```python
from build123d import *

# Parameters (mm, degrees)
SKETCH1_R               = 20
SKETCH1_R_2             = 7.5
BOSS_EXTRUDE1_DEPTH     = 36.5
SKETCH4_R               = 51.5
CUT_EXTRUDE3_DEPTH      = 31.5
CUT_EXTRUDE4_DEPTH      = 247.841548367
CUT_EXTRUDE4_DEPTH_BACK = 247.841548367
SKETCH5_W               = 26.5
SKETCH5_H               = 90
SHELL1_START            = 6
SHELL1_DEPTH            = 30.5
BOSS_EXTRUDE2_START     = -7.5
SKETCH7_R               = 2
BOSS_EXTRUDE2_DEPTH     = 7.5
BOSS_EXTRUDE3_DEPTH     = 15
CUT_EXTRUDE5_DEPTH      = 247.025913269
CUT_EXTRUDE5_DEPTH_BACK = 6
SKETCH9_R               = 5
SKETCH9_R_2             = 1.5
CUT_EXTRUDE6_DEPTH      = 6
FILLET1_R               = 10
SKETCH11_R              = 1.55
CUT_EXTRUDE7_DEPTH      = 247.841548367
SKETCH12_R              = 3.55
CUT_EXTRUDE8_DEPTH      = 3
SKETCH13_R              = 12.1
CUT_EXTRUDE9_DEPTH      = 5


# Read off the part's stored shape, not the designer's step: Shell1
with BuildPart() as part:
    # Sketch1 → Boss-Extrude1 (new body)
    with BuildSketch(Plane.XY):
        with BuildLine():
            ThreePointArc((-54.352625843, 15.42861186), (0, -56.5), (54.352625843, 15.42861186))
            ThreePointArc((54.352625843, 15.42861186), (37.535595393, 105.258460348), (37.34995219, 196.64872093))
            ThreePointArc((37.34995219, 196.64872093), (0, 237.5), (-37.34995219, 196.64872093))
            ThreePointArc((-37.34995219, 196.64872093), (-37.535595393, 105.258460348), (-54.352625843, 15.42861186))
        make_face()
        Circle(SKETCH1_R, mode=Mode.SUBTRACT)
        with Locations((0, 200)):
            Circle(SKETCH1_R_2, mode=Mode.SUBTRACT)
    extrude(amount=BOSS_EXTRUDE1_DEPTH)

    # Sketch4 → Cut-Extrude3 (cut)
    with BuildSketch(Plane.XY.offset(36.5)):
        Circle(SKETCH4_R)
    extrude(amount=-CUT_EXTRUDE3_DEPTH, mode=Mode.SUBTRACT)

    # Sketch5 → Cut-Extrude4 (cut, two sides: drawn at the far end of the back side and taken through both)
    with BuildSketch(Plane(origin=(0, 0, 0), x_dir=(0, 0, -1), z_dir=(1, 0, 0)).offset(-CUT_EXTRUDE4_DEPTH_BACK)):
        with Locations((-23.25, 192.5)):
            Rectangle(SKETCH5_W, SKETCH5_H)
    extrude(amount=CUT_EXTRUDE4_DEPTH + CUT_EXTRUDE4_DEPTH_BACK, mode=Mode.SUBTRACT)

    # Shell1 outline → Shell1 (cut)
    with BuildSketch(Plane.XY.offset(SHELL1_START)):
        with BuildLine():
            ThreePointArc((-42.077009937, 39.188968279), (0, 57.5), (42.077009937, 39.188968279))
            ThreePointArc((42.077009937, 39.188968279), (33.155030313, 90.022278833), (29.457543912, 141.5))
            Line((29.457543912, 141.5), (-29.457543912, 141.5))
            ThreePointArc((-29.457543912, 141.5), (-33.155030313, 90.022278833), (-42.077009937, 39.188968279))
        make_face()
    extrude(amount=SHELL1_DEPTH, mode=Mode.SUBTRACT)

    # Sketch7 → Boss-Extrude2 (add)
    # profile 1 of 2: a face of its own
    with BuildSketch(Plane.XY.offset(36.5).offset(BOSS_EXTRUDE2_START)):
        with BuildLine():
            Line((-39.159181835, 90.358571571), (-46.159181835, 97.5))
            Line((-46.159181835, 97.5), (-46.159181835, 112.5))
            Line((-46.159181835, 112.5), (-36.669554937, 115.653883533))
            ThreePointArc((-36.669554937, 115.653883533), (-37.753606302, 102.990404952), (-39.159181835, 90.358571571))
        make_face()
        with Locations((-42.159181835, 105)):
            Circle(SKETCH7_R, mode=Mode.SUBTRACT)
    # profile 2 of 2: a face of its own
    with BuildSketch(Plane.XY.offset(36.5).offset(BOSS_EXTRUDE2_START)):
        with BuildLine():
            Line((46.159181835, 97.5), (46.159181835, 112.5))
            Line((46.159181835, 112.5), (36.669554937, 115.653883533))
            ThreePointArc((36.669554937, 115.653883533), (37.753606302, 102.990404952), (39.159181835, 90.358571571))
            Line((39.159181835, 90.358571571), (46.159181835, 97.5))
        make_face()
        with Locations(Location((42.159181835, 105, 0), (0, 0, 180))):
            Circle(SKETCH7_R, mode=Mode.SUBTRACT)
    extrude(amount=BOSS_EXTRUDE2_DEPTH)

    # Sketch8 → Boss-Extrude3 (add)
    with BuildSketch(Plane.XY.offset(6)):
        with BuildLine():
            Line((-35.707844492, 72), (-25.707844492, 72))
            Line((-25.707844492, 72), (-25.707844492, 69.5))
            Line((-25.707844492, 69.5), (-36.114376268, 69.5))
            ThreePointArc((-36.114376268, 69.5), (-35.909546125, 70.749745632), (-35.707844492, 72))
        make_face()
        with BuildLine():
            Line((-36.705134195, 66), (-25.707844492, 66))
            Line((-25.707844492, 66), (-25.707844492, 63))
            Line((-25.707844492, 63), (-37.231629056, 63))
            ThreePointArc((-37.231629056, 63), (-36.966124321, 64.499603847), (-36.705134195, 66))
        make_face()
        with BuildLine():
            Line((25.707844492, 63), (37.231629056, 63))
            ThreePointArc((37.231629056, 63), (36.966124321, 64.499603847), (36.705134195, 66))
            Line((36.705134195, 66), (25.707844492, 66))
            Line((25.707844492, 66), (25.707844492, 63))
        make_face()
        with BuildLine():
            Line((25.707844492, 69.5), (36.114376268, 69.5))
            ThreePointArc((36.114376268, 69.5), (35.909546125, 70.749745632), (35.707844492, 72))
            Line((35.707844492, 72), (25.707844492, 72))
            Line((25.707844492, 72), (25.707844492, 69.5))
        make_face()
    extrude(amount=BOSS_EXTRUDE3_DEPTH)

    # Sketch9 → Cut-Extrude5 (cut, two sides: drawn at the far end of the back side and taken through both)
    with BuildSketch(Plane.XY.offset(6).offset(-CUT_EXTRUDE5_DEPTH_BACK)):
        with Locations((0, 90.5)):
            Circle(SKETCH9_R)
        with Locations((-15.5, 106)):
            Circle(SKETCH9_R_2)
        with Locations((15.5, 106)):
            Circle(SKETCH9_R_2)
        with Locations((15.5, 75)):
            Circle(SKETCH9_R_2)
        with Locations((-15.5, 75)):
            Circle(SKETCH9_R_2)
    extrude(amount=CUT_EXTRUDE5_DEPTH + CUT_EXTRUDE5_DEPTH_BACK, mode=Mode.SUBTRACT)

    # Sketch10 → Cut-Extrude6 (cut)
    with BuildSketch(Plane.XY.offset(6)):
        with BuildLine():
            Line((-13.327049627, 124), (-1.672950373, 124))
            ThreePointArc((-1.672950373, 124), (-0.48999582, 123.51000418), (0, 122.327049627))
            Line((0, 122.327049627), (0, 122.172950373))
            ThreePointArc((0, 122.172950373), (-0.48999582, 120.98999582), (-1.672950373, 120.5))
            Line((-1.672950373, 120.5), (-13.327049627, 120.5))
            ThreePointArc((-13.327049627, 120.5), (-14.51000418, 120.98999582), (-15, 122.172950373))
            Line((-15, 122.172950373), (-15, 122.327049627))
            ThreePointArc((-15, 122.327049627), (-14.51000418, 123.51000418), (-13.327049627, 124))
        make_face()
    extrude(amount=-CUT_EXTRUDE6_DEPTH, mode=Mode.SUBTRACT)

    # Fillet1
    fillet1_edges = [part.edges().sort_by_distance(p)[0] for p in [
        (35.369251346, 147.5, 23.25),
        (-35.369251346, 147.5, 23.25),
    ]]
    fillet(fillet1_edges, radius=FILLET1_R)

    # Sketch11 → Cut-Extrude7 (cut, through all)
    with BuildSketch(Plane(origin=(0, 0, 0), x_dir=(-1, 0, 0), z_dir=(0, 0, -1))):
        with Locations((-33.587572106, 33.587572106)):
            Circle(SKETCH11_R)
        with Locations((33.587572106, 33.587572106)):
            Circle(SKETCH11_R)
        with Locations((33.587572106, -33.587572106)):
            Circle(SKETCH11_R)
        with Locations((-33.587572106, -33.587572106)):
            Circle(SKETCH11_R)
    extrude(amount=-CUT_EXTRUDE7_DEPTH, mode=Mode.SUBTRACT)

    # Sketch12 → Cut-Extrude8 (cut)
    with BuildSketch(Plane(origin=(0, 0, 0), x_dir=(-1, 0, 0), z_dir=(0, 0, -1))):
        with Locations((-33.587572106, -33.587572106)):
            Circle(SKETCH12_R)
        with Locations((33.587572106, -33.587572106)):
            Circle(SKETCH12_R)
        with Locations((33.587572106, 33.587572106)):
            Circle(SKETCH12_R)
        with Locations((-33.587572106, 33.587572106)):
            Circle(SKETCH12_R)
    extrude(amount=-CUT_EXTRUDE8_DEPTH, mode=Mode.SUBTRACT)

    # Sketch13 → Cut-Extrude9 (cut)
    with BuildSketch(Plane(origin=(0, 0, 0), x_dir=(-1, 0, 0), z_dir=(0, 0, -1))):
        with Locations((0, 200)):
            Circle(SKETCH13_R)
    extrude(amount=-CUT_EXTRUDE9_DEPTH, mode=Mode.SUBTRACT)


solid = part.part
```
Verification items for the finished model (mm, model axes). A direction names the side the tool comes from. Coordinates: 2 decimals unless noted, no trailing zeros. Order: outer loops, then holes, each group sorted by start corner. A loop starts at its lowest first (then second) coordinate and runs counter-clockwise, first axis right, second up. Notation, with made-up numbers: (35.5, -11) -> (46.5, -11) arc R20 ccw to (46.5, 9) -> close; hole circle Ø8 at (-28, 83). An arc over 180 degrees is marked (long way). Put each result on its own line as item: value. Start each with the question number.
1) Cross-section at C-C (y = 0). Enter the section's corners in (x, z), plus the area to 3 significant figures.
2) Tool access check on faces 4 (the cylindrical face through (-32.602, 144.595, 23.065)), 5 (the cylindrical face through (34.05, -30.068, 1.479)), 6 (the flat face through (-31, 66, 13)). Record the directions out of +Z, -Z, +X, -X, +Y, -Y that give a thin tool (end or side, any length) a straight path to the whole face; none if there is none.
3) Cross-section at B-B (z = 13.5). Enter the section's corners in (x, y) (3 decimals).
4) Cross-section at A-A (y = 200). Enter the section's corners in (x, z), plus the area to 3 significant figures.
5) Release check for a two-part mould opening along X. For faces 1 (the flat face through (40, 103, 29)), 2 (the flat face through (31, 66, 13)), 3 (the flat face through (42.61, 93.88, 32.7)) record: pulls with the +X half, pulls with the -X half, needs draft (parallel to the pull), parting line crosses it, or undercut.
6) Go/stop test with flat-tipped pins: pin 1 (12 mm diameter, centred on y = 43.5, z = 12.5, fed in from +X); pin 2 (24 mm diameter, centred on x = 0, y = 200, fed in from -Z); pin 3 (5 mm diameter, centred on x = 16.5, y = 54, fed in from -Z); pin 4 (2.5 mm diameter, centred on x = -42.16, y = 105, fed in from -Z). Record where each tip stops, or that it passes through.
7) Material ranges on L1, parallel to X at y = 106, z = 1.75; L2, parallel to Y at x = -2.5, z = 18; L3, parallel to Y at x = 10, z = 28.5, recorded low to high.
8) Cross-section at D-D (y = 164). Enter the section's corners in (x, z), plus the area to 3 significant figures.
Geometry check:
1. outline: (-56.5, 0) -> (-20, 0) -> (-20, 5) -> (-51.5, 5) -> (-51.5, 36.5) -> (-56.5, 36.5) -> close; (20, 0) -> (56.5, 0) -> (56.5, 36.5) -> (51.5, 36.5) -> (51.5, 5) -> (20, 5) -> close
1. area: 680 mm^2
2. face 4: +Z, -X, +Y
2. face 5: -Z
2. face 6: +Z
3. outline: (-54.353, 15.429) arc R56.5 ccw (long way) to (54.353, 15.429) arc R500 cw to (35.55, 137.784) arc R10 ccw to (25.554, 147.5) -> (-25.554, 147.5) arc R10 ccw to (-35.55, 137.784) arc R500 cw to start; hole circle Ø103 at (0, 0); hole (-42.077, 39.189) arc R57.5 cw to (42.077, 39.189) arc R506 cw to (37.232, 63) -> (25.708, 63) -> (25.708, 66) -> (36.705, 66) arc R506 cw to (36.114, 69.5) -> (25.708, 69.5) -> (25.708, 72) -> (35.708, 72) arc R506 cw to (29.458, 141.5) -> (-29.458, 141.5) arc R506 cw to (-35.708, 72) -> (-25.708, 72) -> (-25.708, 69.5) -> (-36.114, 69.5) arc R506 cw to (-36.705, 66) -> (-25.708, 66) -> (-25.708, 63) -> (-37.232, 63) arc R506 cw to start
4. outline: (-37.5, 0) -> (-12.1, 0) -> (-12.1, 5) -> (-7.5, 5) -> (-7.5, 10) -> (-37.5, 10) -> close; (7.5, 5) -> (12.1, 5) -> (12.1, 0) -> (37.5, 0) -> (37.5, 10) -> (7.5, 10) -> close
4. area: 554 mm^2
5. face 1: needs draft
5. face 2: undercut
5. face 3: pulls with the +X half
6. pin 1: stops at x = 48.63
6. pin 2: stops at z = 5
6. pin 3: stops at z = 0
6. pin 4: passes through
7. L1: x = -37.47 to -17, -14 to 14, 17 to 37.47
7. L2: y = -56.44 to -51.44, 51.44 to 57.45, 141.5 to 147.5
7. L3: y = -55.61 to -50.52, 50.52 to 56.62, 141.5 to 147.5
8. outline: (-35.49, 0) -> (35.49, 0) -> (35.49, 10) -> (-35.49, 10) -> close
8. area: 710 mm^2
